Part print with two shaded views. Sizes in mm from the minimum x, y, z corner. A direction names the side the tool comes from. Round coordinates to 2 decimals unless told otherwise and drop trailing zeros. Loops run counter-clockwise (first coordinate to the right, second up) from the corner with the lowest first, then second, coordinate; pieces in that order, holes last. Notation, with made-up numbers: (34, -0.5) - (43, -0.5) arc R6 cw to (43, 6.5) - close; hole circle Ø5 at (-33, 44). An arc over 180 degrees is marked (long way). Put each result on its own line as item: value. Start each with the question number.
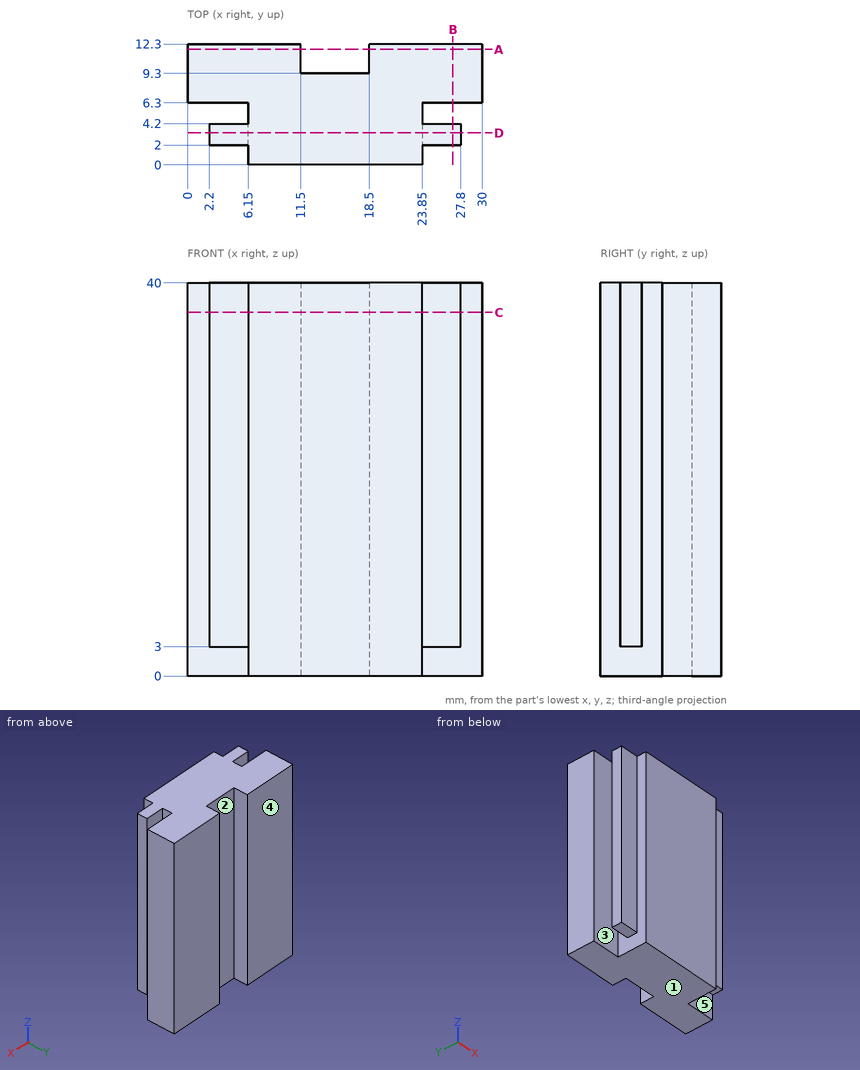
1) Slice it at C-C, the plane z = 37. Write the cut outline in (x, y).
2) Drill centre lines: line 1 (Y direction, x = 4.5, z = 8); line 2 (X direction, y = 11.5, z = 29); line 3 (Y direction, x = 16, z = 26). Where is each one in solid material? Low to high. Write a range as [from, to].
3) Pull direction Y, two halves, no side cores. Call the marked faces 1, 2 and 3: pulls with the +Y half, pulls with the -Y half, needs draft (parallel to the pull), parting line crosses it, or undercut.
4) Slice it at D-D, the plane y = 3.25. Write the cut outline in (x, z), and give its area (3 significant figures).
5) Slice it at A-A, the plane y = 11.75. Write the cut outline in (x, z).
6) Drop flat-ended pins along their axis: pin 1 Ø0.7 at (y, z) = (3, 14.5) entering from +X; pin 2 Ø2.5 at (y, z) = (3, 18.5) entering from -X; pin 3 Ø3 at (x, z) = (27, 24.5) entering from -Y. Give the stop position or say it passes through.
7) Slice it at B-B, the plane x = 27. Write the cut outline in (y, z), and give its area (3 significant figures).
8) Which spindle directions (+Z, -Z, +X, -X, +Y, -Y) get a long thin tool onto all of the face, cutting with end or side? Do the marked faces 4 and 5. Say none if no direction does.
Taken from the geometry:
1. outline: (0, 6.3) - (6.15, 6.3) - (6.15, 4.2) - (2.2, 4.2) - (2.2, 2) - (6.15, 2) - (6.15, 0) - (23.85, 0) - (23.85, 2) - (27.8, 2) - (27.8, 4.2) - (23.85, 4.2) - (23.85, 6.3) - (30, 6.3) - (30, 12.3) - (18.5, 12.3) - (18.5, 9.3) - (11.5, 9.3) - (11.5, 12.3) - (0, 12.3) - close
2. line 1: y = [2, 4.2], [6.3, 12.3]
2. line 2: x = [0, 11.5], [18.5, 30]
2. line 3: y = [0, 9.3]
3. face 1: needs draft
3. face 2: pulls with the +Y half
3. face 3: undercut
4. outline: (2.2, 3) - (6.15, 3) - (6.15, 0) - (23.85, 0) - (23.85, 3) - (27.8, 3) - (27.8, 40) - (2.2, 40) - close
4. area: 1,000 mm2
5. outline: (0, 0) - (11.5, 0) - (11.5, 40) - (0, 40) - close; (18.5, 0) - (30, 0) - (30, 40) - (18.5, 40) - close
6. pin 1: stops at x = 27.8
6. pin 2: stops at x = 2.2
6. pin 3: stops at y = 2
7. outline: (2, 3) - (4.2, 3) - (4.2, 40) - (2, 40) - close; (6.3, 0) - (12.3, 0) - (12.3, 40) - (6.3, 40) - close
7. area: 321 mm2
8. face 4: +Z, -Z, +X, -X, +Y
8. face 5: +Z, -Z, +X
